Build history of the part. All positions in model axes, mm. A direction names the side the tool comes from. Round coordinates to 2 decimals unless told otherwise and drop trailing zeros. Loops run counter-clockwise (first coordinate to the right, second up) from the corner with the lowest first, then second, coordinate; pieces in that order, holes last. Notation, with made-up numbers: (-35, 29.5) - (-3, 29.5) arc R12 cw to (-3, 48.5) - close; hole circle Ø7 at (-17.5, 88). An arc over 180 degrees is marked (long way). Put each result on its own line as item: value. Start each with the question number.
Autodesk Inventor part; units mm, degrees
ref_plane "YZ Plane" through (0, 0, 0) normal (1, 0, 0) x (0, 1, 0)
ref_plane "XZ Plane" through (0, 0, 0) normal (0, 1, 0) x (-1, 0, 0)
ref_plane "XY Plane" through (0, 0, 0) normal (0, 0, 1) x (1, 0, 0)
sketch "Sketch1" plane through (0, 0, 0) normal (0, 0, 1) x (1, 0, 0)
  circle A0 centre (0, 0) radius 3
  circle A1 centre (0, 0) radius 6
  dimension "d0" = 6
  dimension "d1" = 12
extrude "Extrusion1" add sketch "Sketch1" against normal blind 1
sketch "Sketch2" plane through (0, 0, -1) normal (0, 0, -1) x (-1, 0, 0)
  circle A0 centre (0, 0) radius 4
  circle A1 centre (0, 0) radius 3
  dimension "d4" = 8
extrude "Extrusion2" add sketch "Sketch2" along normal blind 5
chamfer "Chamfer1" distance 0.5 angle 45 1 edges at (4, 0, -6)
properties part number "w5f6-12a" material "アセタール樹脂、黒"
Item 1: Slice it at D-D (y = -5). Give the cut face in (x, z).
Item 2: Drill centre lines: probe 1 along Y at (x, z) = (0, -3.1); probe 2 along Z at (x, y) = (0.75, 5.5); probe 3 along X at (y, z) = (0.75, -2.65). Where is each one in solid material? Low to high. Write a range as [from, to].
Item 3: Which spindle directions (+Z, -Z, +X, -X, +Y, -Y) get a long thin tool onto all of the face, cutting with end or side? Do faces 1 (the flat face through (-1.42, -3.92, -1)), 2 (the flat face through (-3, -1, 0)). Say none if no direction does.
Item 4: Slice it at A-A (x = 0). Give the cut face in (y, z), plus the area to 4 significant figures.
Item 5: Slice it at C-C (z = -0.8). Give the cut face in (x, y), plus the area to 3 significant figures.
Item 6: Drop a flat-ended pin along its axis: pin 1 Ø2 at (y, z) = (-2, -1.5) entering from -X. Give the stop position or say it passes through.
Computed values:
1. outline: (-3.32, -1) - (3.32, -1) - (3.32, 0) - (-3.32, 0) - close
2. probe 1: y = [-4, -3], [3, 4]
2. probe 2: z = [-1, 0]
2. probe 3: x = [-3.93, -2.9], [2.9, 3.93]
3. face 1: -Z
3. face 2: +Z, +X, -X, +Y, -Y
4. outline: (-6, -1) - (-4, -1) - (-4, -5.5) - (-3.5, -6) - (-3, -6) - (-3, 0) - (-6, 0) - close; (3, -6) - (3.5, -6) - (4, -5.5) - (4, -1) - (6, -1) - (6, 0) - (3, 0) - close
4. area: 15.75 mm^2
5. outline: circle Ø12 at (0, 0); hole circle Ø6 at (0, 0)
5. area: 84.8 mm^2
6. pin 1: stops at x = -5.89
